For this review, use the dimensioned drawing (mm, ordinates from the lowest corner) and the shaded views. Round coordinates to 2 decimals unless told otherwise and drop trailing zeros. Order: outer loops, then holes, each group sorted by start corner. A loop starts at its lowest first (then second) coordinate and runs counter-clockwise, first axis right, second up. Notation, with made-up numbers: M 81,-23 L 111,-23 A10 ccw 111,-6 Z; hole C 2,54 d6. An arc over 180 degrees is marked long. Put each result on its own line as item: value.
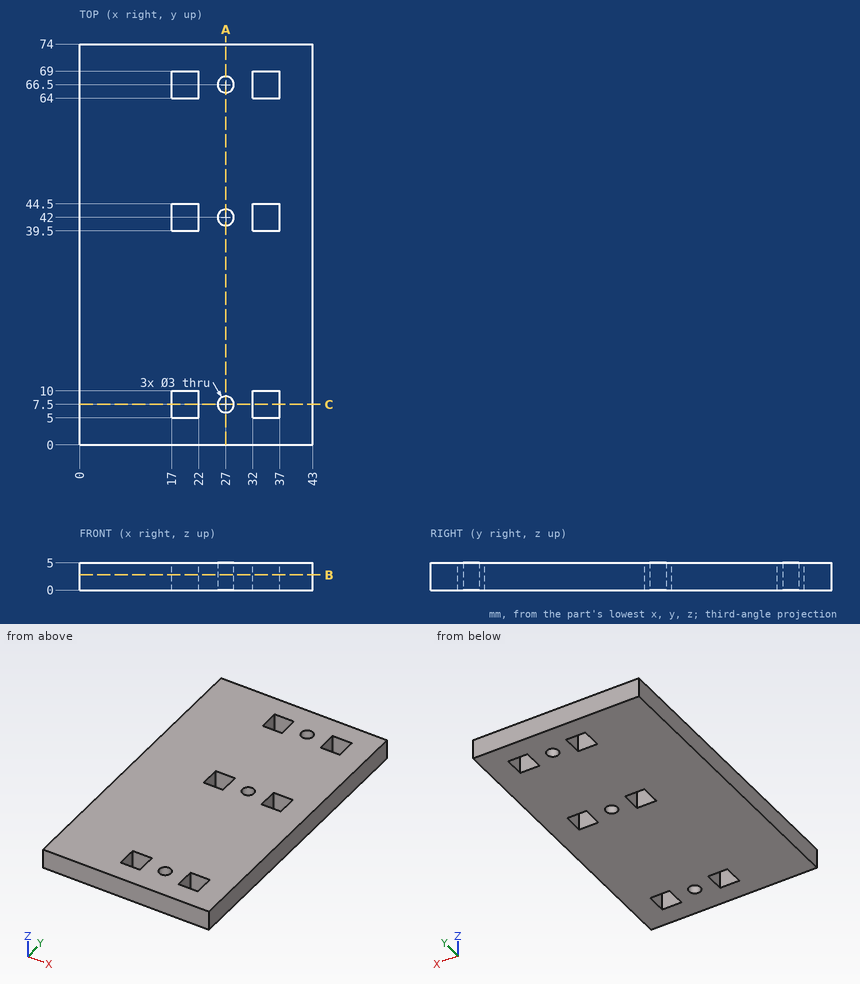
(1) Add section C-C on y = 7.5. Give the boundary of the cut face in (x, z), then the cut area to 3 significant figures.
A:
outline: M 0,0 L 17,0 L 17,5 L 0,5 Z; M 22,0 L 25.5,0 L 25.5,5 L 22,5 Z; M 28.5,0 L 32,0 L 32,5 L 28.5,5 Z; M 37,0 L 43,0 L 43,5 L 37,5 Z
area: 150 mm2
(2) Add section A-A on x = 27. Give the boundary of the cut face in (y, z).
A:
outline: M 0,0 L 6,0 L 6,5 L 0,5 Z; M 9,0 L 40.5,0 L 40.5,5 L 9,5 Z; M 43.5,0 L 65,0 L 65,5 L 43.5,5 Z; M 68,0 L 74,0 L 74,5 L 68,5 Z
(3) To check wall thickness, follow L1, parallel to Y at x = 27, z = 2.75; L2, parallel to Y at x = 17.5, z = 2.3. State the ranges of each line that lie inside material, in increasing order.
A:
L1: y = 0 to 6, 9 to 40.5, 43.5 to 65, 68 to 74
L2: y = 0 to 5, 10 to 39.5, 44.5 to 64, 69 to 74
(4) Add section B-B on z = 2.8. State how many separate pieces and enclosed holes the cut face has, then the cut area to 3 significant figures.
A:
separate pieces: 1
enclosed holes: 9
area: 3,010 mm2
